Check sheet for the modelled part. Datum: model origin and axes. Units: mm. Coordinates: 2 decimals unless noted, no trailing zeros. Order: outer loops, then holes, each group sorted by start corner. A loop starts at its lowest first (then second) coordinate and runs counter-clockwise, first axis right, second up.
from build123d import *

# Parameters (mm, degrees)
F4_DEPTH = 30
F5_R     = 10
F6_DEPTH = 60


with BuildPart() as f2:
    # F0 (on Top) → F2 (revolve)
    with BuildSketch(Plane.XY):
        with BuildLine():
            Line((0, -30), (0, 30))
            ThreePointArc((0, 30), (-30, 0), (0, -30))
        make_face()
    revolve(axis=Axis((0, 0, 0), (0, -1, 0)))

    # F3 (on Front) → F4 (cut, symmetric)
    with BuildSketch(Plane.XZ):
        with BuildLine():
            Line((30, 0), (-30, 0))
            ThreePointArc((-30, 0), (0, -30), (30, 0))
        make_face()
    extrude(amount=F4_DEPTH, both=True, mode=Mode.SUBTRACT)

    # F5 (on face) → F6 (cut)
    with BuildSketch(Plane(origin=(0, 0, 0), x_dir=(1, 0, 0), z_dir=(0, 0, -1))):
        Circle(F5_R)
    extrude(amount=-F6_DEPTH, mode=Mode.SUBTRACT)


solid = f2.part
(1) Cross-section at C-C (z = 19.75). Enter the section's corners in (x, y).
Filled in:
outline: circle Ø45.16 at (0, 0); hole circle Ø20 at (0, 0)
(2) Go/stop test with flat-tipped pins: P1, Ø5, axis at x = -21.5, z = 13, coming from the +Y side; P2, Ø10, axis at x = 0, z = 19, coming from the -Y side; P3, Ø18, axis at x = 0, y = 0, coming from the +Z side; P4, Ø6, axis at x = -18.5, y = -4.5, coming from the +Z side. Record where each tip stops, or that it passes through.
Filled in:
P1: stops at y = 19.7
P2: stops at y = -26.53
P3: passes through
P4: stops at z = 25.35
(3) Release check for a two-part mould opening along X. For faces 1 (the flat face through (0, 13, 0)), 2 (the cylindrical face through (-2.17, 9.76, 13.94)) record: +X half, -X half, draft (parallel to the pull), parting line (faces both ways), or undercut.
Filled in:
face 1: draft
face 2: undercut
(4) Cross-section at A-A (y = 0). Enter the section's corners in (x, z).
Filled in:
outline: (-30, 0) - (-10, 0) - (-10, 28.28) arc R30 ccw to start; (10, 0) - (30, 0) arc R30 ccw to (10, 28.28) - close
(5) Thickness scan on probe 1 along Y at (x, z) = (7, 19); probe 2 along Y at (x, z) = (0, 8); probe 3 along X at (y, z) = (3, 12.75). Record the ranges inside material, lowest first.
Filled in:
probe 1: y = -22.14 to -7.14, 7.14 to 22.14
probe 2: y = -28.91 to -10, 10 to 28.91
probe 3: x = -26.99 to -9.54, 9.54 to 26.99
(6) Cross-section at D-D (x = 25.5). Enter the section's corners in (y, z).
Filled in:
outline: (-15.8, 0) - (15.8, 0) arc R15.8 ccw to start
